The listing builds one solid part. Answer for the finished solid, in the listing's coordinates (mm). A direction names the side the tool comes from. Round coordinates to 2 decimals unless told otherwise and drop trailing zeros. Loops run counter-clockwise (first coordinate to the right, second up) from the corner with the lowest first, then second, coordinate; pieces in that order, holes last. Notation, with made-up numbers: (8.5, -8) - (45.5, -8) arc R18 ccw to (45.5, 27) - close; hole circle Ø2 at (34.5, 9). An arc over 180 degrees is marked (long way). Write item = value, one per line. Start each with the question number.
1) Given pin 1 Ø2 at (y, z) = (-3, -2) entering from +X; pin 2 Ø1.5 at (y, z) = (-4.5, -2.5) entering from -X; pin 3 Ø2 at (x, z) = (4, 2) entering from -Y, each flat-ended and moving along its own axis, determine where each tip first touches the part or whether it passes through.
2) For a pull along X with two mould halves and no side action, classify faces 1 (the cylindrical face through (11.207, 3.529, -0.035)), 2 (the cylindrical face through (0.342, 17.497, 3.993)), 3 (the cylindrical face through (-11.43, -6.85, 1.3)), 4 (the flat face through (-4.1, -10.4, -3.5)) as released by +X, released by -X, zero draft, split by the parting line, or undercut.
3) A tool of negligible diameter and unlimited length cuts with its end or side. For faces 5 (the cylindrical face through (-15.6, 1.2, 4)), 6 (the cylindrical face through (-3.27, -14.74, 0.54)), 7 (the cylindrical face through (15.6, -1.2, 4)), 8 (the cylindrical face through (-0.342, -17.497, 3.993)), 9 (the flat face through (-2, 10, -2.5)), from which of +Z, -Z, +X, -X, +Y, -Y can it reach the whole face along a straight path? Write none if from no direction.
4) Section B-B, the plane z = 0.25 is taken. Determine the outline of the cut face in (x, y), and give its area (3 significant figures).
5) Straight lines are drawn through the part: line 1 along Y through (x, z) = (0, 0.75); line 2 along Z through (x, y) = (-5.5, 14.5); line 3 along X through (y, z) = (-3.5, 0.5). For each, find the intervals that lie inside material, in ascending order.
6) Section A-A, the plane x = 0 is taken. Give the number of separate pieces and of enclosed holes in the cut face, and give its area (3 significant figures).
from build123d import *

# Parameters (mm, degrees)
SKETCH_1_R               = 15.1
SKETCH_1_R_2             = 11.750000000000002
EXTRUDE_1_DEPTH          = 3.5
SKETCH_2_R               = 11.750000000000004
SKETCH_2_R_2             = 9.750000000000002
EXTRUDE_2_DEPTH          = 1
FILLET_1_R               = 1
FILLET_2_R               = 1
SKETCH_3_R               = 17.500000000000004
SKETCH_3_R_2             = 11.750000000000002
EXTRUDE_3_DEPTH          = 1
CUT_EXTRUDE_1_DEPTH      = 26.719642299223374
FILLET_3_R               = 2
FILLET_4_R               = 1
SKETCH_6_R               = 1.0000000000000007
CUT_EXTRUDE_2_DEPTH      = 6.5
PATTERN_CIRCULAR_2_COUNT = 3
FILLET_6_R               = 0.5
CHAMFER_1_SIZE           = 0.4
CHAMFER_1_SIZE2          = 2


# Some blends are built 0.0001 mm under size
with BuildPart() as part:
    # 草图1 → 凸台-拉伸1 (new, symmetric)
    with BuildSketch(Plane.XY):
        Circle(SKETCH_1_R)
        Circle(SKETCH_1_R_2, mode=Mode.SUBTRACT)
    extrude(amount=EXTRUDE_1_DEPTH, both=True)

    # 草图2 → 凸台-拉伸2 (add)
    with BuildSketch(Plane(origin=(0, 0, -3.5), x_dir=(-1, 0, 0), z_dir=(0, 0, -1))):
        Circle(SKETCH_2_R)
        Circle(SKETCH_2_R_2, mode=Mode.SUBTRACT)
    extrude(amount=-EXTRUDE_2_DEPTH)

    # 圆角1
    fillet_1_edges = [part.edges().sort_by_distance(p)[0] for p in [
        (-15.1, 1.85e-15, -3.5),
    ]]
    fillet(fillet_1_edges, radius=FILLET_1_R)

    # 圆角2
    fillet_2_edges = [part.edges().sort_by_distance(p)[0] for p in [
        (9.750000000000002, 1.19e-15, -3.5),
    ]]
    fillet(fillet_2_edges, radius=FILLET_2_R - 0.0001)  # a hair under: the kernel refuses the full size

    # 草图3 → 凸台-拉伸3 (add)
    with BuildSketch(Plane.XY.offset(3.5)):
        Circle(SKETCH_3_R)
        with Locations(Location((0, 0, 0), (0, 0, 180))):
            Circle(SKETCH_3_R_2, mode=Mode.SUBTRACT)
    extrude(amount=EXTRUDE_3_DEPTH)

    # 草图4 → 切除-拉伸1 (cut, through all)
    with BuildSketch(Plane(origin=(0, 0, 3.5), x_dir=(-1, 0, 0), z_dir=(0, 0, -1))):
        with BuildLine():
            Line((-20.056660766424834, 2), (-15.06784656146989, 2))
            ThreePointArc((-15.06784656146989, 2), (-15.2, 1.86e-15), (-15.06784656146989, -2))
            Line((-15.06784656146989, -2), (-20.056660766424834, -2))
            Line((-20.056660766424834, -2), (-20.056660766424834, 2))
        make_face()
    cut_extrude_1 = extrude(amount=-CUT_EXTRUDE_1_DEPTH, mode=Mode.SUBTRACT)

    # 镜向1: 切除-拉伸1 across plane
    add(cut_extrude_1.mirror(Plane(origin=(0, 0, 0), x_dir=(0, 0, 1), z_dir=(1, 0, 0))), mode=Mode.SUBTRACT)

    # 圆角3
    fillet_3_edges = [part.edges().sort_by_distance(p)[0] for p in [
        (-15.067846561469892, -2, 4),
        (-15.067846561469892, 2, 4),
        (15.067846561469892, -2, 4),
        (15.067846561469892, 2, 4),
    ]]
    fillet(fillet_3_edges, radius=FILLET_3_R - 0.0001)  # a hair under: the kernel refuses the full size

    # 圆角4
    fillet_4_edges = [part.edges().sort_by_distance(p)[0] for p in [
        (17.385338650713713, 2, 4),
        (17.385338650713713, -2, 4),
        (-17.385338650713713, -2, 4),
        (-17.385338650713713, 2, 4),
    ]]
    fillet(fillet_4_edges, radius=FILLET_4_R)

    # 草图6 → 切除-拉伸2 (cut)
    with BuildSketch(Plane.XY.offset(4.500000000000001)):
        with Locations((7.1e-16, 14.299999999999999)):
            Circle(SKETCH_6_R)
    cut_extrude_2 = extrude(amount=-CUT_EXTRUDE_2_DEPTH, mode=Mode.SUBTRACT)

    # 阵列(圆周)2: 切除-拉伸2 ×3 about axis
    pattern_circular_2_axis = Axis((6.2e-16, -9.3e-16, 0), (0, 0, 1))
    for i in range(1, PATTERN_CIRCULAR_2_COUNT):
        add(cut_extrude_2.rotate(pattern_circular_2_axis, i * 360 / PATTERN_CIRCULAR_2_COUNT), mode=Mode.SUBTRACT)

    # 圆角6
    # the kernel refuses this fillet: 0.5 mm, written as the material it takes off along each edge
    with BuildSketch(Plane(origin=(-0.6164263274586522, 15.087412587412588, -1.9999999999999991), x_dir=(-0.9974594960272485, -0.0712359023601691, 0), z_dir=(0, 0, 1))) as fillet_6_piece_1:
        with BuildLine():
            CenterArc((0.9045816644890499, 0.49976803448578755), FILLET_6_R, 167.30835919933298, 104.43698518013807)
            ThreePointArc((0.41679836041578583, 0.6096199724175768), (0.2667346233621471, 0.2649259303036035), (0, 0))
            ThreePointArc((0, 0), (0.4599051560196865, -0.00700535852919151), (0.9198103120393711, 0))
        make_face()
    extrude(amount=5.499999999999999, mode=Mode.SUBTRACT)
    with BuildSketch(Plane(origin=(0.6164263274586537, 15.087412587412588, -1.9999999999999991), x_dir=(0.9974594960272485, -0.0712359023601691, 0), z_dir=(0, 0, 1))) as fillet_6_piece_2:
        with BuildLine():
            CenterArc((0.90458166448905, -0.49976803448578755), FILLET_6_R, 88.25465562052895, 104.43698518013832)
            ThreePointArc((0.41679836041578633, -0.6096199724175786), (0.266734623362148, -0.26492593030360523), (0, 0))
            ThreePointArc((0, 0), (0.45990515601968684, 0.00700535852919153), (0.9198103120393712, 0))
        make_face()
    extrude(amount=5.499999999999999, mode=Mode.SUBTRACT)
    with BuildSketch(Plane(origin=(13.374295741805769, -7.00986543456549, -1.9999999999999991), x_dir=(0.4370376469082089, 0.8994432139857056, 0), z_dir=(0, 0, 1))) as fillet_6_piece_3:
        with BuildLine():
            CenterArc((0.9045816644889654, 0.4997680344857882), FILLET_6_R, 167.30835919933284, 104.4369851801381)
            ThreePointArc((0.41679836041570123, 0.6096199724175785), (0.2667346233620795, 0.26492593030362477), (0, 0))
            ThreePointArc((0, 0), (0.45990515601963466, -0.00700535852919092), (0.9198103120392858, 0))
        make_face()
    extrude(amount=5.499999999999999, mode=Mode.SUBTRACT)
    with BuildSketch(Plane(origin=(12.757869414347034, -8.077547152847108, -1.9999999999999991), x_dir=(-0.5604218491190406, -0.8282073116255346, 0), z_dir=(0, 0, 1))) as fillet_6_piece_4:
        with BuildLine():
            CenterArc((0.9045816644889654, -0.49976803448578744), FILLET_6_R, 88.25465562052915, 104.43698518013807)
            ThreePointArc((0.4167983604157008, -0.6096199724175783), (0.26673462336207926, -0.264925930303624), (0, 0))
            ThreePointArc((0, 0), (0.4599051560196484, 0.00700535852919206), (0.9198103120392849, 3e-17))
        make_face()
    extrude(amount=5.499999999999999, mode=Mode.SUBTRACT)
    with BuildSketch(Plane(origin=(-12.757869414347084, -8.07754715284703, -1.9999999999999991), x_dir=(0.5604218491190395, -0.8282073116255352, 0), z_dir=(0, 0, 1))) as fillet_6_piece_5:
        with BuildLine():
            CenterArc((0.9045816644890518, 0.4997680344857874), FILLET_6_R, 167.30835919933295, 104.43698518013798)
            ThreePointArc((0.4167983604157886, 0.6096199724175766), (0.26673462336214776, 0.26492593030360556), (0, 0))
            ThreePointArc((0, 0), (0.4599051560196818, -0.00700535852919271), (0.9198103120393719, 3e-17))
        make_face()
    extrude(amount=5.499999999999999, mode=Mode.SUBTRACT)
    with BuildSketch(Plane(origin=(-13.374295741805737, -7.009865434565554, -1.9999999999999991), x_dir=(-0.43703764690820945, 0.8994432139857054, 0), z_dir=(0, 0, 1))) as fillet_6_piece_6:
        with BuildLine():
            CenterArc((0.9045816644890493, -0.4997680344857882), FILLET_6_R, 88.25465562052901, 104.43698518013812)
            ThreePointArc((0.4167983604157851, -0.6096199724175783), (0.2667346233621474, -0.26492593030360473), (0, 0))
            ThreePointArc((0, 0), (0.4599051560196919, 0.00700535852919249), (0.91981031203937, 2e-17))
        make_face()
    extrude(amount=5.499999999999999, mode=Mode.SUBTRACT)

    # 倒角1
    chamfer_1_edges = [part.edges().sort_by_distance(p)[0] for p in [
        (11.750000000000002, -8.1e-15, 4.5),
    ]]
    chamfer_1_side = [part.faces().sort_by_distance(p)[0] for p in [
        (15.179125181594527, 1.457318687256729, 4.5),
    ]]
    chamfer(chamfer_1_edges, length=CHAMFER_1_SIZE, length2=CHAMFER_1_SIZE2, reference=chamfer_1_side[0])


solid = part.part
Geometry check:
q1.pin_1 = 14.97
q1.pin_2 = -14.63
q1.pin_3 = -14.8
q2.face_1 = undercut
q2.face_2 = split by the parting line
q2.face_3 = undercut
q2.face_4 = zero draft
q3.face_5 = +Z, -Z, -X
q3.face_6 = -Z
q3.face_7 = +Z, -Z, +X
q3.face_8 = +Z, -Z, -Y
q3.face_9 = +Z
q4.outline = (-13.78, -6.18) arc R0.5 ccw to (-13.01, -6.37) arc R1 cw (long way) to (-12.02, -8.08) arc R0.5 ccw to (-12.24, -8.84) arc R15.1 ccw to (12.24, -8.84) arc R0.5 ccw to (12.02, -8.08) arc R1 cw (long way) to (13.01, -6.37) arc R0.5 ccw to (13.78, -6.18) arc R15.1 ccw to (1.53, 15.02) arc R0.5 ccw to (0.99, 14.45) arc R1 cw (long way) to (-0.99, 14.45) arc R0.5 ccw to (-1.53, 15.02) arc R15.1 ccw to start; hole circle Ø23.5 at (0, 0)
q4.area = 273 mm2
q5.line_1 = -15.1 to -11.75, 11.75 to 13.3
q5.line_2 = 3.5 to 4.5
q5.line_3 = -14.69 to -11.22, 11.22 to 14.69
q6.separate_pieces = 3
q6.enclosed_holes = 0
q6.area = 48.8 mm2
